Read the model definition and answer for the solid it produces. Units are mm, in the model's axes. Face numbers are marked on the shaded views. A direction names the side the tool comes from. Coordinates: 2 decimals unless noted, no trailing zeros. Order: outer loops, then holes, each group sorted by start corner. A loop starts at its lowest first (then second) coordinate and runs counter-clockwise, first axis right, second up. Notation, with made-up numbers: (-20.75, 6) - (-4.75, 6) arc R11 ccw to (-4.75, 26) - close; hole circle Ø10 at (74.5, -26). An arc over 180 degrees is marked (long way). Use one line per item in the form item = value. Start each with the question number.
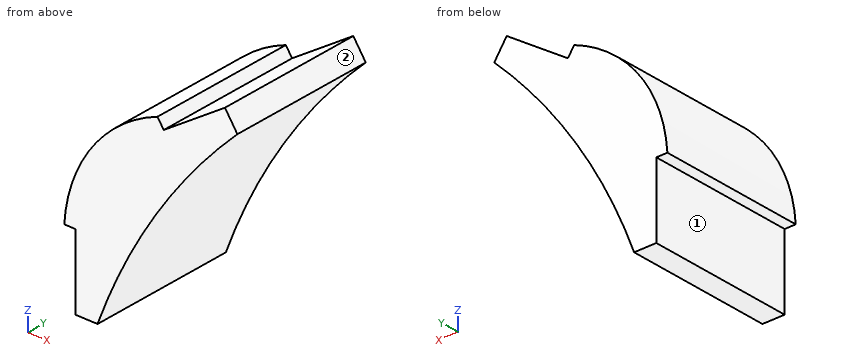
Autodesk Fusion 360 part; units mm, degrees
sketch "Rear Most Corner" plane through (0, 0, 0) normal (0, 1, 0) x (1, 0, 0)
  circle A0 centre (23.1977, -483.5644) radius 25 construction
  line L0 (14.257, -506.911) -> (24.7715, -514.0339) construction
  line L1 (407.957, -773.6165) -> (14.257, -506.911) construction
  line L2 (-1.7526, -485.14) -> (-1.7526, -472.44) construction
  line L3 (24.7715, -514.0339) -> (14.257, -506.911) construction
  line L4 (14.257, -506.911) -> (15.3255, -505.3338)
  line L5 (15.3255, -505.3338) -> (25.84, -512.4567)
  line L6 (25.84, -512.4567) -> (24.7715, -514.0339) construction
  line L7 (-1.7526, -485.14) -> (0.1524, -485.14)
  line L8 (0.1524, -485.14) -> (0.1524, -472.44)
  line L9 (0.1524, -472.44) -> (-1.7526, -472.44) construction
  line L10 (-1.7526, -472.44) -> (-1.7526, -485.14) construction
  line L11 (-1.7526, -485.14) -> (0.1524, -485.14)
  line L12 (14.257, -506.911) -> (15.3255, -505.3338)
  arc A1 (-1.7526, -485.14) -> (14.257, -506.911) centre (23.1977, -483.5644) ccw
  line L13 (25.84, -512.4567) -> (27.9768, -509.3024)
  line L14 (0.1524, -472.44) -> (3.9624, -472.44)
  line L15 (3.0571, -498.3751) -> (23.1977, -483.5644) construction
  arc A2 (3.9624, -472.44) -> (27.9768, -509.3024) centre (97.8219, -437.5475) ccw
  point P0 (13.1274, -490.9697)
extrude "Extrude1" add sketch "Rear Most Corner" along normal blind 25.4
Q1. A cutting plane is placed at A-A (y = 10). Give the vertices of the cut face in (x, z), then the cut area to 3 significant figures.
Q2. A cutting plane is placed at B-B (z = 495). Give the vertices of the cut face in (x, y), then the cut area to 3 significant figures.
Q3. Consider probe 1 along X at (y, z) = (18.75, 487.5); probe 2 along X at (y, z) = (24.25, 503); probe 3 along Z at (x, y) = (18, 24.25). Determine where each line is inside the solid, lowest interval first.
Q4. Given P1, Ø1, axis at x = 22, y = 11, coming from the +Z side; P2, Ø1, axis at x = -0.5, y = 14.5, coming from the -Z side; P3, Ø3, axis at x = 2.5, y = 8.5, coming from the +Z side, each flat-ended and moving along its own axis, determine where each tip first touches the part or whether it passes through.
Q5. A cutting plane is placed at C-C (x = 12.75). Give the vertices of the cut face in (y, z), then the cut area to 3 significant figures.
Q6. Which of the six approach directions +Z, -Z, +X, -X, +Y, -Y give full straight-line access (tool end or side, diameter ignored) to the marked faces 1 and 2?
Result sheet:
q1.outline = (-1.75, 485.14) - (0.15, 485.14) - (0.15, 472.44) - (3.96, 472.44) arc R100.14 cw to (27.98, 509.3) - (25.84, 512.46) - (15.33, 505.33) - (14.26, 506.91) arc R25 ccw to start
q1.area = 413 mm^2
q2.outline = (0.97, 0) - (15.81, 0) - (15.81, 25.4) - (0.97, 25.4) - close
q2.area = 377 mm^2
q3.probe_1 = -1.49 to 11.04
q3.probe_2 = 7.47 to 22.04
q3.probe_3 = 498.01 to 507.15
q4.P1 = 510.19
q4.P2 = 485.14
q4.P3 = 499.58
q5.outline = (0, 490.37) - (25.4, 490.37) - (25.4, 506.28) - (0, 506.28) - close
q5.area = 404 mm^2
q6.face_1 = -Z, -X, +Y, -Y
q6.face_2 = +Z, +X, +Y, -Y
